Geometry check sheet. Reference: the model listing, model coordinates, mm. A direction names the side the tool comes from. Round coordinates to 2 decimals unless told otherwise and drop trailing zeros. Order: outer loops, then holes, each group sorted by start corner. A loop starts at its lowest first (then second) coordinate and runs counter-clockwise, first axis right, second up. Notation, with made-up numbers: M -36,31 L -26,31 A33 cw -26,61 Z; hole C 89,13.25 d10. An arc over 180 degrees is marked long. Return JSON: item names as keys, results as strings. Group by question number.
```python
from build123d import *

# Parameters (mm, degrees)
SALIENTE_EXTRUIR1_DEPTH = 20
CROQUIS2_W              = 20
CROQUIS2_H              = 23
CORTAR_EXTRUIR1_DEPTH   = 101.09995005
CORTAR_EXTRUIR3_DEPTH   = 18


with BuildPart() as part:
    # Croquis1 → Saliente-Extruir1 (new, symmetric)
    with BuildSketch(Plane(origin=(0, 0, 0), x_dir=(0, 0, -1), z_dir=(1, 0, 0))):
        Polygon((0, 0), (-94, 0), (-94, 18), (-64, 18), (-64, 46), (-30, 46), (-30, 18), (0, 18), align=None)
    extrude(amount=SALIENTE_EXTRUIR1_DEPTH, both=True)

    # Croquis2 → Cortar-Extruir1 (cut, through all)
    with BuildSketch(Plane(origin=(0, 18, 0), x_dir=(1, 0, 0), z_dir=(0, 1, 0))):
        with Locations((0, -82.5)):
            Rectangle(CROQUIS2_W, CROQUIS2_H)
        with Locations((0, -11.5)):
            Rectangle(CROQUIS2_W, CROQUIS2_H)
    extrude(amount=-CORTAR_EXTRUIR1_DEPTH, mode=Mode.SUBTRACT)

    # Croquis3 → Cortar-Extruir3 (cut)
    with BuildSketch(Plane(origin=(0, 46, 0), x_dir=(1, 0, 0), z_dir=(0, 1, 0))):
        with BuildLine():
            Line((5, -59), (5, -64))
            Line((5, -64), (-5, -64))
            Line((-5, -64), (-5, -59))
            ThreePointArc((-5, -59), (-13, -47), (-5, -35))
            Line((-5, -35), (-5, -30))
            Line((-5, -30), (5, -30))
            Line((5, -30), (5, -35))
            ThreePointArc((5, -35), (13, -47), (5, -59))
        make_face()
    extrude(amount=-CORTAR_EXTRUIR3_DEPTH, mode=Mode.SUBTRACT)


solid = part.part
```
Q1. Material ranges on line 1 along X through (y, z) = (13, 20); line 2 along Z through (x, y) = (-8, 20); line 3 along Y through (x, z) = (7, 37), recorded low to high.
Q2. Set-up check for faces 1 (the face through (0, 9, 23)), 2 (the face through (-5, 37, 62)), 3 (the face through (0, 9, 71)), 4 (the face through (13, 37, 47)), 5 (the face through (0, 18, 69)): record each of +Z, -Z, +X, -X, +Y, -Y from which the full face is reachable in a straight line by a thin tool's end or side.
Q3. Release check for a two-part mould opening along Z. For faces 6 (the face through (0, 28, 47)), 7 (the face through (10, 9, 83)), 8 (the face through (-15, 9, 0)) record: +Z half, -Z half, draft (parallel to the pull), parting line (faces both ways), or undercut.
Q4. Section check B-B on z = 8. Record the cut outline in (x, y), plus the area to 3 significant figures.
Q5. Depth check by flat-ended pin: pin 1 Ø14 at (x, y) = (1.5, 29.5) entering from +Z; pin 2 Ø22.5 at (x, y) = (4.5, 38.5) entering from -Z; pin 3 Ø9 at (x, y) = (0.5, 9) entering from +Z; pin 4 Ø3 at (x, z) = (-11, 53) entering from +Y. Enter the tip coordinate at first touch or a pass-through.
Q6. Section check A-A on y = 40.5. Record the cut outline in (x, z).
Q7. Section check C-C on x = -3.5. Record the cut outline in (y, z).
Q8. Section check D-D on z = 32. Record the cut outline in (x, y), plus the area to 3 significant figures.
Geometry check:
{
 "1": {"line 1": "x = -20 to -10, 10 to 20", "line 2": "z = 30 to 64", "line 3": "y = 0 to 28"},
 "2": {"face 1": "-Z, +Y, -Y", "face 2": "+Z, -Z, +Y", "face 3": "+Z, +Y, -Y", "face 4": "+Y", "face 5": "+Z, +X, -X, +Y"},
 "3": {"face 6": "undercut", "face 7": "draft", "face 8": "-Z half"},
 "4": {"outline": "M -20,0 L -10,0 L -10,18 L -20,18 Z; M 10,0 L 20,0 L 20,18 L 10,18 Z", "area": "360 mm^2"},
 "5": {"pin 1": "stops at z = 64", "pin 2": "stops at z = 30", "pin 3": "stops at z = 71", "pin 4": "stops at y = 46"},
 "6": {"outline": "M -20,30 L -5,30 L -5,35 A13 cw -5,59 L -5,64 L -20,64 Z; M 5,30 L 20,30 L 20,64 L 5,64 L 5,59 A13 cw 5,35 Z"},
 "7": {"outline": "M 0,23 L 18,23 L 18,30 L 28,30 L 28,64 L 18,64 L 18,71 L 0,71 Z"},
 "8": {"outline": "M -20,0 L 20,0 L 20,46 L 5,46 L 5,28 L -5,28 L -5,46 L -20,46 Z", "area": "1,660 mm^2"}
}
